```python
from build123d import *

# Parameters (mm, degrees)
BOSS_EXTRUDE1_DEPTH = 431.8
SKETCH2_R           = 5.207
CUT_EXTRUDE1_DEPTH  = 25.4


with BuildPart() as part:
    # Sketch1 → Boss-Extrude1 (new body)
    with BuildSketch(Plane(origin=(0, 0, 0), x_dir=(1, 0, 0), z_dir=(0, 1, 0))):
        with BuildLine():
            Line((-25.4, 0), (25.4, 0))
            ThreePointArc((25.4, 0), (0, 25.4), (-25.4, 0))
        make_face()
    extrude(amount=BOSS_EXTRUDE1_DEPTH)

    # Sketch2 → Cut-Extrude1 (cut)
    with BuildSketch(Plane(origin=(0, 431.8, 0), x_dir=(1, 0, 0), z_dir=(0, 1, 0))):
        with Locations(Location((-11.54495024, 9.057446198, 0), (0, 0, 270))):
            Circle(SKETCH2_R)
        with Locations(Location((11.54495024, 9.057446198, 0), (0, 0, 270))):
            Circle(SKETCH2_R)
    extrude(amount=-CUT_EXTRUDE1_DEPTH, mode=Mode.SUBTRACT)


solid = part.part
```
Here's how the part is built. I have some questions about the finished solid (model axes, mm). A direction names the side the tool comes from. Give positions to 0.01 mm unless a question says otherwise; leave off trailing zeros. Loops run counter-clockwise (first coordinate to the right, second up) from the corner with the lowest first, then second, coordinate; pieces in that order, holes last. Notation, with made-up numbers: M 84,-36.75 L 114,-36.75 A15 ccw 114,-14.75 Z; hole C 49,9.5 d3. An arc over 180 degrees is marked long. Use one line per item in the form item = value. Start each with the question number.
Q1. Thinking about a two-plate mould opening in Z: for faces 1 (the cylindrical face through (0.559, 212.877, -25.394)), 2 (the flat face through (0, 0, -10)), 3 (the flat face through (-11, 406.4, -9)), 4 (the flat face through (0, 213, 0)), which applies, +Z half, -Z half, draft (parallel to the pull), parting line (faces both ways), or undercut?
Q2. Which directions (+Z, -Z, +X, -X, +Y, -Y) give clear straight access to the entire face, cutting with the end or side of a thin tool? Please do faces 5 (the cylindrical face through (8.38, 419.28, -13.19)), 6 (the flat face through (0, 431.8, -10)).
Q3. Will these pins go through, and if not, where does the flat tip stop? pin 1 Ø5 at (x, y) = (17, 119) entering from -Z; pin 2 Ø2 at (y, z) = (52.5, -3.5) entering from -X; pin 3 Ø8.5 at (x, z) = (11.54, -9.06) entering from +Y.
Q4. If we section it at A-A (z = -8.25): Write out the boundary of the cut face in (x, y).
Q5. If we section it at B-B (y = 115.5): Write out the boundary of the cut face in (x, z).
Q6. I need wall thicknesses on line 1 along X through (y, z) = (407, -12.5); line 2 along Y through (x, z) = (11, -12.25); line 3 along X through (y, z) = (122, -22.5). Which ranges of each line are inside material? Lowest first, please.
Taken from the geometry:
q1.face_1 = -Z half
q1.face_2 = draft
q1.face_3 = undercut
q1.face_4 = +Z half
q2.face_5 = +Y
q2.face_6 = +Z, -Z, +X, -X, +Y
q3.pin_1 = -20.85
q3.pin_2 = -25.28
q3.pin_3 = 406.4
q4.outline = M -24.02,0 L 24.02,0 L 24.02,431.8 L 16.69,431.8 L 16.69,406.4 L 6.4,406.4 L 6.4,431.8 L -6.4,431.8 L -6.4,406.4 L -16.69,406.4 L -16.69,431.8 L -24.02,431.8 Z
q5.outline = M -25.4,0 A25.4 ccw 25.4,0 Z
q6.line_1 = -22.11 to -15.45, -7.64 to 7.64, 15.45 to 22.11
q6.line_2 = 0 to 406.4
q6.line_3 = -11.79 to 11.79
